```python
from build123d import *

# Parameters (mm, degrees)
SKETCH1_W            = 326
SKETCH1_H            = 117.8
SKETCH1_W_2          = 318.2
SKETCH1_H_2          = 110
BOSS_EXTRUDE1_DEPTH  = 20
SKETCH1_3_W          = 318.2
SKETCH1_3_H          = 110
BOSS_EXTRUDE2_DEPTH  = 3
BOSS_EXTRUDE6_START  = 3
SKETCH6_R            = 3.25
SKETCH6_R_2          = 1.8
BOSS_EXTRUDE6_DEPTH  = 3.2
FILLET1_R            = 22
CUT_EXTRUDE3_START   = 163
CUT_EXTRUDE3_DEPTH   = 3.9
CUT_EXTRUDE4_START   = 1.2
SKETCH6_2_R          = 1.8
CUT_EXTRUDE4_DEPTH   = 1.8
SKETCH5_W            = 64.404478897
SKETCH5_H            = 11.204693833
SKETCH5_W_2          = 4
SKETCH5_H_2          = 98.795306167
SKETCH5_W_3          = 30.218685567
SKETCH5_H_3          = 8.375486052
SKETCH5_H_4          = 73.388395798
SKETCH5_W_4          = 147.589311785
SKETCH5_H_5          = 5.740206696
BOSS_EXTRUDE7_DEPTH  = 14.4
CUT_EXTRUDE5_START   = -58.9
SKETCH10_R           = 6.5
CUT_EXTRUDE5_DEPTH   = 3.9
BOSS_EXTRUDE8_START  = -55
SKETCH11_W           = 18
SKETCH11_H           = 2.429995135
SKETCH11_W_2         = 3
SKETCH11_H_2         = 3
BOSS_EXTRUDE8_DEPTH  = 3.3
BOSS_EXTRUDE9_START  = -51.7
BOSS_EXTRUDE9_DEPTH  = 3
BOSS_EXTRUDE10_START = 3
SKETCH12_R           = 3
BOSS_EXTRUDE10_DEPTH = 17
SKETCH12_3_R         = 3
CUT_EXTRUDE6_DEPTH   = 6
SKETCH13_R           = 4.5
CUT_EXTRUDE7_DEPTH   = 4


with BuildPart() as part:
    # Sketch1 → Boss-Extrude1 (new body)
    with BuildSketch(Plane.XY):
        Rectangle(SKETCH1_W, SKETCH1_H)
        Rectangle(SKETCH1_W_2, SKETCH1_H_2, mode=Mode.SUBTRACT)
    extrude(amount=BOSS_EXTRUDE1_DEPTH)

    # Sketch1<3> → Boss-Extrude2 (add)
    with BuildSketch(Plane.XY):
        Rectangle(SKETCH1_3_W, SKETCH1_3_H)
    extrude(amount=BOSS_EXTRUDE2_DEPTH)

    # Sketch6 → Boss-Extrude6 (add)
    # profile 1 of 4: a face of its own
    with BuildSketch(Plane.XY.offset(BOSS_EXTRUDE6_START)):
        with Locations((132, -24.5)):
            Circle(SKETCH6_R)
        with Locations((132, -24.5)):
            Circle(SKETCH6_R_2, mode=Mode.SUBTRACT)
    # profile 2 of 4: a face of its own
    with BuildSketch(Plane.XY.offset(BOSS_EXTRUDE6_START)):
        with Locations((74, -24.5)):
            Circle(SKETCH6_R)
        with Locations((74, -24.5)):
            Circle(SKETCH6_R_2, mode=Mode.SUBTRACT)
    # profile 3 of 4: a face of its own
    with BuildSketch(Plane.XY.offset(BOSS_EXTRUDE6_START)):
        with Locations((74, 24.5)):
            Circle(SKETCH6_R)
        with Locations((74, 24.5)):
            Circle(SKETCH6_R_2, mode=Mode.SUBTRACT)
    # profile 4 of 4: a face of its own
    with BuildSketch(Plane.XY.offset(BOSS_EXTRUDE6_START)):
        with Locations((132, 24.5)):
            Circle(SKETCH6_R)
        with Locations((132, 24.5)):
            Circle(SKETCH6_R_2, mode=Mode.SUBTRACT)
    extrude(amount=BOSS_EXTRUDE6_DEPTH)

    # Fillet1
    fillet1_edges = [part.edges().sort_by_distance(p)[0] for p in [
        (163, 58.9, 10),
        (163, -58.9, 10),
        (-163, -58.9, 10),
        (-163, 58.9, 10),
        (159.1, 55, 11.5),
        (-159.1, 55, 11.5),
        (-159.1, -55, 11.5),
        (159.1, -55, 11.5),
    ]]
    fillet(fillet1_edges, radius=FILLET1_R)

    # Sketch9 → Cut-Extrude3 (cut)
    with BuildSketch(Plane(origin=(0, 0, 0), x_dir=(0, 0, -1), z_dir=(1, 0, 0)).offset(CUT_EXTRUDE3_START)):
        with BuildLine():
            Line((-20, -8.55), (-8.58, -8.55))
            ThreePointArc((-8.58, -8.55), (-8.226446609, -8.403553391), (-8.08, -8.05))
            Line((-8.08, -8.05), (-8.08, 6.05))
            ThreePointArc((-8.08, 6.05), (-8.226446609, 6.403553391), (-8.58, 6.55))
            Line((-8.58, 6.55), (-20, 6.55))
            Line((-20, 6.55), (-20, -8.55))
        make_face()
    extrude(amount=-CUT_EXTRUDE3_DEPTH, mode=Mode.SUBTRACT)

    # Sketch6<2> → Cut-Extrude4 (cut)
    with BuildSketch(Plane.XY.offset(CUT_EXTRUDE4_START)):
        with Locations((132, -24.5)):
            Circle(SKETCH6_2_R)
        with Locations((132, 24.5)):
            Circle(SKETCH6_2_R)
        with Locations((74, 24.5)):
            Circle(SKETCH6_2_R)
        with Locations((74, -24.5)):
            Circle(SKETCH6_2_R)
    extrude(amount=CUT_EXTRUDE4_DEPTH, mode=Mode.SUBTRACT)

    # Sketch5 → Boss-Extrude7 (add)
    with BuildSketch(Plane.XY):
        with Locations((-66.797760552, 49.397653084)):
            Rectangle(SKETCH5_W, SKETCH5_H)
        with Locations((-101, 5.602346917)):
            Rectangle(SKETCH5_W_2, SKETCH5_H_2)
        with Locations((48.890657217, 50.812256974)):
            Rectangle(SKETCH5_W_3, SKETCH5_H_3)
        with Locations((66, 49.397653084)):
            Rectangle(SKETCH5_W_2, SKETCH5_H)
        with Locations((66, 0)):
            Rectangle(SKETCH5_W_2, SKETCH5_H_4)
        with Locations((-9.794655893, -52.129896652)):
            Rectangle(SKETCH5_W_4, SKETCH5_H_5)
        with Locations((66, -49.397653084)):
            Rectangle(SKETCH5_W_2, SKETCH5_H)
    extrude(amount=BOSS_EXTRUDE7_DEPTH)

    # Sketch10 → Cut-Extrude5 (cut)
    with BuildSketch(Plane(origin=(0, 0, 0), x_dir=(1, 0, 0), z_dir=(0, 1, 0)).offset(CUT_EXTRUDE5_START)):
        with Locations((95, -16.665643961)):
            Circle(SKETCH10_R)
        with Locations((-95, -16.665643961)):
            Circle(SKETCH10_R)
    extrude(amount=CUT_EXTRUDE5_DEPTH, mode=Mode.SUBTRACT)

    # Sketch11 → Boss-Extrude8 (add)
    with BuildSketch(Plane(origin=(0, 0, 0), x_dir=(1, 0, 0), z_dir=(0, 1, 0)).offset(BOSS_EXTRUDE8_START)):
        Polygon((-104.033941149, -14.931036323), (-101.03394878, -14.937802738), (-101.040715195, -17.937795107), (-104.040707565, -17.931028692), align=None)
        Polygon((-86.018356525, -8.041657306), (-104.018310741, -8.001058815), (-104.023791526, -10.431047769), (-86.023837311, -10.47164626), align=None)
        with Locations((95, -9.450646394)):
            Rectangle(SKETCH11_W, SKETCH11_H)
        with Locations((102.5, -16.665643961)):
            Rectangle(SKETCH11_W_2, SKETCH11_H_2)
    extrude(amount=BOSS_EXTRUDE8_DEPTH)

    # Sketch11<3> → Boss-Extrude9 (add)
    with BuildSketch(Plane(origin=(0, 0, 0), x_dir=(1, 0, 0), z_dir=(0, 1, 0)).offset(BOSS_EXTRUDE9_START)):
        Polygon((86, -8.235648826), (86, -10.665643961), (91, -10.665643961), (91, -20), (99, -20), (99, -10.665643961), (104, -10.665643961), (104, -8.235648826), align=None)
        Polygon((-104.023791526, -10.431047769), (-99.023804244, -10.442325128), (-99.044857621, -19.776657424), (-91.044877969, -19.794701198), (-91.023824593, -10.460368902), (-86.023837311, -10.47164626), (-86.018356525, -8.041657306), (-104.018310741, -8.001058815), align=None)
    extrude(amount=BOSS_EXTRUDE9_DEPTH)

    # Sketch12 → Boss-Extrude10 (add)
    # profile 1 of 4: a face of its own
    with BuildSketch(Plane.XY.offset(BOSS_EXTRUDE10_START)):
        with BuildLine():
            Line((-137.1, -55), (-137.1, -48))
            ThreePointArc((-137.1, -48), (-141.493398282, -37.393398282), (-152.1, -33))
            Line((-152.1, -33), (-159.1, -33))
            ThreePointArc((-159.1, -33), (-152.656349186, -48.556349186), (-137.1, -55))
        make_face()
        with Locations((-146.828174593, -42.728174593)):
            Circle(SKETCH12_R, mode=Mode.SUBTRACT)
    # profile 2 of 4: a face of its own
    with BuildSketch(Plane.XY.offset(BOSS_EXTRUDE10_START)):
        with BuildLine():
            ThreePointArc((-137.1, 48), (-141.493398282, 37.393398282), (-152.1, 33))
            Line((-152.1, 33), (-159.1, 33))
            ThreePointArc((-159.1, 33), (-152.656349186, 48.556349186), (-137.1, 55))
            Line((-137.1, 55), (-137.1, 48))
        make_face()
        with Locations((-146.828174593, 42.728174593)):
            Circle(SKETCH12_R, mode=Mode.SUBTRACT)
    # profile 3 of 4: a face of its own
    with BuildSketch(Plane.XY.offset(BOSS_EXTRUDE10_START)):
        with BuildLine():
            ThreePointArc((152.1, 33), (141.493398282, 37.393398282), (137.1, 48))
            Line((137.1, 48), (137.1, 55))
            ThreePointArc((137.1, 55), (152.656349186, 48.556349186), (159.1, 33))
            Line((159.1, 33), (152.1, 33))
        make_face()
        with Locations((146.828174593, 42.728174593)):
            Circle(SKETCH12_R, mode=Mode.SUBTRACT)
    # profile 4 of 4: a face of its own
    with BuildSketch(Plane.XY.offset(BOSS_EXTRUDE10_START)):
        with BuildLine():
            ThreePointArc((137.1, -48), (141.493398282, -37.393398282), (152.1, -33))
            Line((152.1, -33), (159.1, -33))
            ThreePointArc((159.1, -33), (152.656349186, -48.556349186), (137.1, -55))
            Line((137.1, -55), (137.1, -48))
        make_face()
        with Locations((146.828174593, -42.728174593)):
            Circle(SKETCH12_R, mode=Mode.SUBTRACT)
    extrude(amount=BOSS_EXTRUDE10_DEPTH)

    # Sketch12<3> → Cut-Extrude6 (cut)
    with BuildSketch(Plane.XY):
        with Locations((146.828174593, 42.728174593)):
            Circle(SKETCH12_3_R)
        with Locations((146.828174593, -42.728174593)):
            Circle(SKETCH12_3_R)
        with Locations((-146.828174593, -42.728174593)):
            Circle(SKETCH12_3_R)
        with Locations((-146.828174593, 42.728174593)):
            Circle(SKETCH12_3_R)
    extrude(amount=CUT_EXTRUDE6_DEPTH, mode=Mode.SUBTRACT)

    # Sketch13 → Cut-Extrude7 (cut)
    with BuildSketch(Plane.XY):
        with Locations((-146.828174593, -42.728174593)):
            Circle(SKETCH13_R)
        with Locations((-146.828174593, 42.728174593)):
            Circle(SKETCH13_R)
        with Locations((146.828174593, 42.728174593)):
            Circle(SKETCH13_R)
        with Locations((146.828174593, -42.728174593)):
            Circle(SKETCH13_R)
    extrude(amount=CUT_EXTRUDE7_DEPTH, mode=Mode.SUBTRACT)


solid = part.part
```
Geometry: final body of the model. Coordinates: model frame, mm. A direction names the side the tool comes from. Round coordinates to 2 decimals unless told otherwise and drop trailing zeros. Write each loop counter-clockwise with the first axis right and the second up, starting at its lowest first coordinate (ties: lowest second). Pieces come first, ordered by that corner, then holes. Notation, with made-up numbers: (28.25, 76) -> (48.25, 76) arc R5 cw to (48.25, 84) -> close; hole circle Ø1 at (61.5, 41.5). An arc over 180 degrees is marked (long way). Use CSV: the item, a comma, the result in double quotes. Start each with the question number.
Q1. Section B-B (x = 25.5). Return loops of the section in (y, z), plus the area to 3 significant figures.
Q2. Line query: L1, parallel to X at y = 18, z = 12.75; L2, parallel to Y at x = 132, z = 3.7; L3, parallel to X at y = 6, z = 8.25. Output: solid intervals per line, ascending.
Q3. Section A-A (x = 120). Return loops of the section in (y, z).
Q4. Pull-direction query (X, two-part tool) for faces 6 (the face through (-2, -58.9, 10)), 7 (the face through (75.4, 23.1, 6.2)); classes: pulls with the +X half, pulls with the -X half, needs draft (parallel to the pull), parting line crosses it, or undercut.
Q5. Reachability of faces 1 (the face through (144.62, -40.7, 11.89)), 2 (the face through (148, -46, 4)), 3 (the face through (95, -52, 8.236)), 4 (the face through (-94.81, -56.98, 10.17)), 5 (the face through (-141.38, -37.51, 11.38)) from +Z, -Z, +X, -X, +Y, -Y: full face, straight path, thin tool, end or side. Return the list, or none.
Q6. First-contact query: pin 1 Ø1.2 at (y, z) = (-51.5, 9.5) entering from +X; pin 2 Ø8 at (x, y) = (-146.83, -42.73) entering from -Z; pin 3 Ø2 at (y, z) = (-53, 13) entering from -X. Flat tips, straight axial feed; report the tip coordinate or a pass-through.
Result sheet:
1,outline,"(-58.9, 0) -> (58.9, 0) -> (58.9, 20) -> (55, 20) -> (55, 3) -> (-49.26, 3) -> (-49.26, 14.4) -> (-55, 14.4) -> (-55, 20) -> (-58.9, 20) -> close"
1,area,"551 mm²"
2,L1,"-163 to -159.1, -103 to -99, 64 to 68, 159.1 to 163"
2,L2,"-58.9 to -55, -27.75 to -26.3, -22.7 to -21.25, 21.25 to 22.7, 26.3 to 27.75, 55 to 58.9"
2,L3,"-163 to -159.1, -103 to -99, 64 to 68"
3,outline,"(-58.9, 0) -> (58.9, 0) -> (58.9, 20) -> (55, 20) -> (55, 3) -> (-55, 3) -> (-55, 20) -> (-58.9, 20) -> close"
4,face 6,"needs draft"
4,face 7,"undercut"
5,face 1,"+Z, -Z"
5,face 2,"-Z"
5,face 3,"none"
5,face 4,"-Y"
5,face 5,"+Z"
6,pin 1,"x = 157.97"
6,pin 2,"z = 4"
6,pin 3,"x = -157"
